Source: CAD feature listing. Evaluate the final solid. Frame: model axes, mm. Face numbers are marked on the shaded views. A direction names the side the tool comes from. Give positions to 0.01 mm unless a question says otherwise; leave off trailing zeros. Loops run counter-clockwise (first coordinate to the right, second up) from the corner with the lowest first, then second, coordinate; pieces in that order, holes last. Notation, with made-up numbers: M 11,21.5 L 70,21.5 A10 ccw 70,38.5 Z; hole C -2,-14 d9. An arc over 180 degrees is marked long. Answer in a Markdown table with one row per item.
```python
from build123d import *

# Parameters (mm, degrees)
F0_W     = 127
F0_H     = 50.8
F3_DEPTH = 25.4
F4_W     = 25.4
F4_H     = 101.6
F5_DEPTH = 152.401
F6_R     = 12.7
F7_DEPTH = 152.401


with BuildPart() as f1:
    # F0 (on Front) → F1 (revolve)
    with BuildSketch(Plane.XZ):
        with Locations((63.5, 25.4)):
            Rectangle(F0_W, F0_H)
    revolve(axis=Axis((0, 0, 25.4), (0, 0, 1)))

    # F2 (on Right) → F3 (join, symmetric)
    with BuildSketch(Plane.YZ):
        with BuildLine():
            Line((-25.4, 88.9), (-25.4, 50.8))
            Line((-25.4, 50.8), (25.4, 50.8))
            Line((25.4, 50.8), (25.4, 88.9))
            ThreePointArc((25.4, 88.9), (0, 114.3), (-25.4, 88.9))
        make_face()
    extrude(amount=F3_DEPTH, both=True)

    # F4 (on face) → F5 (cut, through all)
    with BuildSketch(Plane(origin=(0, 25.4, 0), x_dir=(-1, 0, 0), z_dir=(0, 1, 0))):
        with Locations((0, 101.6)):
            Rectangle(F4_W, F4_H)
    extrude(amount=-F5_DEPTH, mode=Mode.SUBTRACT)

    # F6 (on face) → F7 (cut, through all)
    with BuildSketch(Plane.YZ.offset(25.4)):
        with Locations((0, 88.9)):
            Circle(F6_R)
    extrude(amount=-F7_DEPTH, mode=Mode.SUBTRACT)


solid = f1.part
```
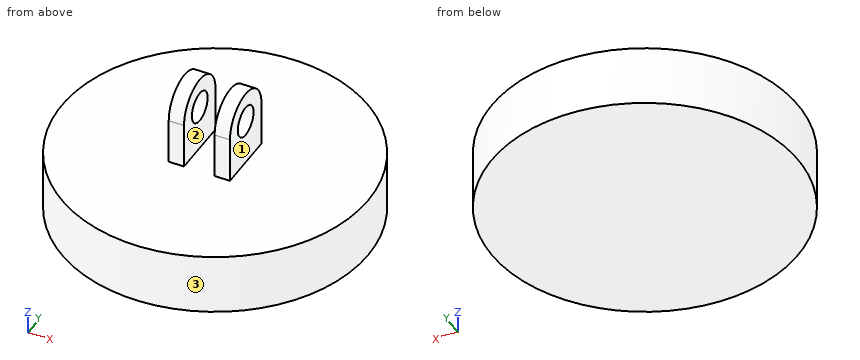
1) Section A-A, the plane y = 0. Return loops of the section in (x, z).
Reply:
| item | result |
|---|---|
| outline | M -127,0 L 127,0 L 127,50.8 L 25.4,50.8 L 25.4,76.2 L 12.7,76.2 L 12.7,50.8 L -12.7,50.8 L -12.7,76.2 L -25.4,76.2 L -25.4,50.8 L -127,50.8 Z; M -25.4,101.6 L -12.7,101.6 L -12.7,114.3 L -25.4,114.3 Z; M 12.7,101.6 L 25.4,101.6 L 25.4,114.3 L 12.7,114.3 Z |
2) Material intervals for L1, parallel to Z at x = 15.75, y = 0; L2, parallel to X at y = -20.5, z = 61.5; L3, parallel to Z at x = 39, y = -97, sorted ascending.
Reply:
| item | result |
|---|---|
| L1 | z = 0 to 76.2, 101.6 to 114.3 |
| L2 | x = -25.4 to -12.7, 12.7 to 25.4 |
| L3 | z = 0 to 50.8 |
3) Set-up query: the marked faces 1, 2 and 3. Return all of +Z, -Z, +X, -X, +Y, -Y with unobstructed straight access to the full face (end or side cutting, diameter ignored); none if empty.
Reply:
| item | result |
|---|---|
| face 1 | +Z, +X, +Y, -Y |
| face 2 | +Z, +Y, -Y |
| face 3 | +Z, -Z |
4) Section C-C, the plane z = 84.5. Return loops of the section in (x, y).
Reply:
| item | result |
|---|---|
| outline | M -25.4,-25.4 L -12.7,-25.4 L -12.7,-11.91 L -25.4,-11.91 Z; M -25.4,11.91 L -12.7,11.91 L -12.7,25.4 L -25.4,25.4 Z; M 12.7,-25.4 L 25.4,-25.4 L 25.4,-11.91 L 12.7,-11.91 Z; M 12.7,11.91 L 25.4,11.91 L 25.4,25.4 L 12.7,25.4 Z |
5) Pin query (flat end, axial travel): pin 1 Ø12 at (x, z) = (71, 39) entering from +Y; pin 2 Ø4 at (y, z) = (-21, 80) entering from -X; pin 3 Ø10 at (x, z) = (18.5, 79) entering from +Y. Return the tip coordinate at first contact, or that it passes through.
Reply:
| item | result |
|---|---|
| pin 1 | stops at y = 109.11 |
| pin 2 | stops at x = -25.4 |
| pin 3 | stops at y = 25.4 |
6) Section B-B, the plane z = 54. Return loops of the section in (x, y), then the cut area to 3 significant figures.
Reply:
| item | result |
|---|---|
| outline | M -25.4,-25.4 L -12.7,-25.4 L -12.7,25.4 L -25.4,25.4 Z; M 12.7,-25.4 L 25.4,-25.4 L 25.4,25.4 L 12.7,25.4 Z |
| area | 1,290 mm² |
7) Section D-D, the plane x = 0. Return loops of the section in (y, z), then the cut area to 3 significant figures.
Reply:
| item | result |
|---|---|
| outline | M -127,0 L 127,0 L 127,50.8 L -127,50.8 Z |
| area | 12,900 mm² |
